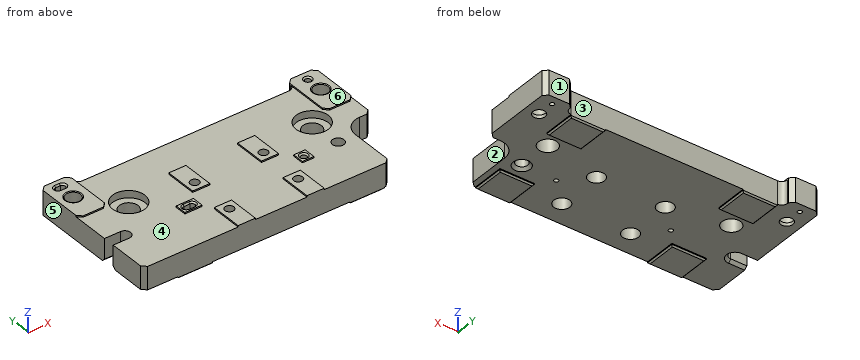
from build123d import *

# Parameters (mm, degrees)
SKETCH1_W                                        = 152.4
SKETCH1_H                                        = 69.85
BASE_EXTRUDE_DEPTH                               = 12.7
SKETCH29_W                                       = 19.05
SKETCH29_H                                       = 17.78
MOUNTING_SURFACES_STAGE2_DEPTH                   = 1.27
CHAMFER1_SIZE                                    = 2.286
SKETCH17_W                                       = 9.525
SKETCH17_H                                       = 17.4625
MOUNTING_SURFACES_MAGNET_BRACKET_DEPTH           = 0.762
EXTRUDE1_DEPTH                                   = 13.462
SKETCH18_R                                       = 1.59512
PIN_HOLES_SLOTS_MAGNET_BLOCK_BOBIN_DEPTH         = 1.762
PIN_HOLES_SLOTS_MAGNET_BLOCK_BOBIN_DEPTH_BACK    = 6.35
SKETCH19_W                                       = 6.35
SKETCH19_H                                       = 6.35
SKETCH19_R                                       = 1.59512
SKETCH19_W_2                                     = 9.525
PIN_HOLE_SLOT_MAGNET_BLOCK_SURFACE_DEPTH         = 0.762
CLEARANCE_CUT_GS_13_SCREW_HEAD_DEPTH             = 1.762
CLEARANCE_CUT_GS_13_SCREW_HEAD_DEPTH_BACK        = 14.97
CBORE_FOR_8_SOCKET_HEAD_CAP_SCREW1_D             = 4.9149
CBORE_FOR_8_SOCKET_HEAD_CAP_SCREW1_CBORE_D       = 8.89
CBORE_FOR_8_SOCKET_HEAD_CAP_SCREW1_CBORE_DEPTH   = 7.62
TAPPED_HOLE_FOR_1_4_20_HELICOIL1_AT_2_COUNT      = 2
TAPPED_HOLE_FOR_1_4_20_HELICOIL1_AT_2_PITCH      = 137.16
SKETCH28_R                                       = 3.18389
PIN_HOLE_SLOT_TO_STAGE2_DEPTH                    = 15.732
CBORE_FOR_3_8_SOCKET_HEAD_CAP_SCREW1_D           = 10.3124
CBORE_FOR_3_8_SOCKET_HEAD_CAP_SCREW1_CBORE_D     = 17.8562
CBORE_FOR_3_8_SOCKET_HEAD_CAP_SCREW1_CBORE_DEPTH = 3.9624
CHAMFER3_SIZE                                    = 0.762
F_3_32_0_09375_DIAMETER_HOLE1_D                  = 2.38125
CHAMFER4_SIZE                                    = 1.524
SKETCH37_W                                       = 15.875
SKETCH37_H                                       = 6.0325
EXTRUDE2_DEPTH                                   = 0.762
FILLET1_R                                        = 3.175
CHAMFER7_SIZE                                    = 0.762
CHAMFER8_SIZE                                    = 2.286


with BuildPart() as part:
    # Sketch1 → Base Extrude (new body)
    with BuildSketch(Plane.XY):
        with Locations((0, 9.525)):
            Rectangle(SKETCH1_W, SKETCH1_H)
    extrude(amount=BASE_EXTRUDE_DEPTH)

    # Sketch29 → Mounting Surfaces_ Stage2 (add)
    with BuildSketch(Plane(origin=(0, 0, 0), x_dir=(-1, 0, 0), z_dir=(0, 0, -1))):
        with Locations((-47.625, 35.56)):
            Rectangle(SKETCH29_W, SKETCH29_H)
        with Locations((-47.625, -16.51)):
            Rectangle(SKETCH29_W, SKETCH29_H)
        with Locations((47.625, 35.56)):
            Rectangle(SKETCH29_W, SKETCH29_H)
        with Locations((47.625, -16.51)):
            Rectangle(SKETCH29_W, SKETCH29_H)
    extrude(amount=MOUNTING_SURFACES_STAGE2_DEPTH)

    # Chamfer1
    chamfer1_edges = [part.edges().sort_by_distance(p)[0] for p in [
        (-76.2, 44.45, 6.35),
        (76.2, 44.45, 6.35),
        (76.2, -25.4, 6.35),
        (-76.2, -25.4, 6.35),
    ]]
    chamfer(chamfer1_edges, length=CHAMFER1_SIZE)

    # Sketch17 → Mounting Surfaces_ Magnet _ Bracket (add)
    with BuildSketch(Plane.XY.offset(12.7)):
        with Locations((-19.05, 16.66875)):
            Rectangle(SKETCH17_W, SKETCH17_H)
        with Locations((19.05, 16.66875)):
            Rectangle(SKETCH17_W, SKETCH17_H)
        with Locations((19.05, -16.66875)):
            Rectangle(SKETCH17_W, SKETCH17_H)
        with Locations((-19.05, -16.66875)):
            Rectangle(SKETCH17_W, SKETCH17_H)
        Polygon((-73.914, 44.45), (-76.2, 42.164), (-76.2, 27.94), (-60.325, 27.94), (-60.325, 44.45), align=None)
        Polygon((73.914, 44.45), (60.325, 44.45), (60.325, 27.94), (76.2, 27.94), (76.2, 42.164), align=None)
    extrude(amount=MOUNTING_SURFACES_MAGNET_BRACKET_DEPTH)

    # Sketch36 → Extrude1 (add)
    with BuildSketch(Plane.XY.offset(13.462)):
        Polygon((-76.2, 42.164), (-76.2, 48.1965), (-73.914, 50.4825), (-60.325, 50.4825), (-60.325, 44.45), (-73.914, 44.45), align=None)
        Polygon((60.325, 44.45), (60.325, 50.4825), (73.914, 50.4825), (76.2, 48.1965), (76.2, 42.164), (73.914, 44.45), align=None)
    extrude(amount=-EXTRUDE1_DEPTH)

    # Sketch18 → Pin holes _ Slots_ Magnet Block _ Bobin (cut, two sides)
    with BuildSketch(Plane.XY.offset(12.7)) as pin_holes_slots_magnet_block_bobin_sk:
        with Locations((31.75, 0)):
            Circle(SKETCH18_R)
        with Locations((68.58, 45.72)):
            Circle(SKETCH18_R)
        with BuildLine():
            Line((-33.3375, 1.59512), (-30.1625, 1.59512))
            ThreePointArc((-30.1625, 1.59512), (-28.56738, 0), (-30.1625, -1.59512))
            Line((-30.1625, -1.59512), (-33.3375, -1.59512))
            ThreePointArc((-33.3375, -1.59512), (-34.93262, 0), (-33.3375, 1.59512))
        make_face()
        with BuildLine():
            Line((-69.85, 47.31512), (-67.31, 47.31512))
            ThreePointArc((-67.31, 47.31512), (-65.71488, 45.72), (-67.31, 44.12488))
            Line((-67.31, 44.12488), (-69.85, 44.12488))
            ThreePointArc((-69.85, 44.12488), (-71.44512, 45.72), (-69.85, 47.31512))
        make_face()
    extrude(amount=PIN_HOLES_SLOTS_MAGNET_BLOCK_BOBIN_DEPTH, mode=Mode.SUBTRACT)
    extrude(pin_holes_slots_magnet_block_bobin_sk.sketch, amount=-PIN_HOLES_SLOTS_MAGNET_BLOCK_BOBIN_DEPTH_BACK, mode=Mode.SUBTRACT)

    # Sketch19 → Pin hole _ Slot_ Magnet Block surface (add)
    with BuildSketch(Plane.XY.offset(12.7)):
        with Locations((31.75, 0)):
            Rectangle(SKETCH19_W, SKETCH19_H)
        with Locations((31.75, 0)):
            Circle(SKETCH19_R, mode=Mode.SUBTRACT)
        with Locations((-31.75, 0)):
            Rectangle(SKETCH19_W_2, SKETCH19_H)
        with BuildLine():
            Line((-30.1625, 1.59512), (-33.3375, 1.59512))
            ThreePointArc((-33.3375, 1.59512), (-34.93262, 0), (-33.3375, -1.59512))
            Line((-33.3375, -1.59512), (-30.1625, -1.59512))
            ThreePointArc((-30.1625, -1.59512), (-28.56738, 0), (-30.1625, 1.59512))
        make_face(mode=Mode.SUBTRACT)
    extrude(amount=PIN_HOLE_SLOT_MAGNET_BLOCK_SURFACE_DEPTH)

    # Sketch20 → Clearance Cut_ GS-13 Screw Head (cut, two sides)
    with BuildSketch(Plane.XY.offset(12.7)) as clearance_cut_gs_13_screw_head_sk:
        with BuildLine():
            Line((60.325, 0), (60.325, -25.4))
            Line((60.325, -25.4), (73.914, -25.4))
            Line((73.914, -25.4), (76.2, -23.114))
            Line((76.2, -23.114), (76.2, 9.525))
            Line((76.2, 9.525), (69.85, 9.525))
            ThreePointArc((69.85, 9.525), (63.114807909, 6.735192091), (60.325, 0))
        make_face()
    extrude(amount=CLEARANCE_CUT_GS_13_SCREW_HEAD_DEPTH, mode=Mode.SUBTRACT)
    extrude(clearance_cut_gs_13_screw_head_sk.sketch, amount=-CLEARANCE_CUT_GS_13_SCREW_HEAD_DEPTH_BACK, mode=Mode.SUBTRACT)

    # CBORE for _8 Socket Head Cap Screw1 (through all)
    with Locations(Plane(origin=(0, 0, 0), x_dir=(-1, 0, 0), z_dir=(0, 0, -1))):
        with Locations((-19.05, 12.7), (19.05, 12.7), (19.05, -12.7), (-19.05, -12.7)):
            CounterBoreHole(CBORE_FOR_8_SOCKET_HEAD_CAP_SCREW1_D / 2, CBORE_FOR_8_SOCKET_HEAD_CAP_SCREW1_CBORE_D / 2, CBORE_FOR_8_SOCKET_HEAD_CAP_SCREW1_CBORE_DEPTH)

    # Sketch25 → Tapped Hole for 1_4-20 Helicoil1 (revolve, cut)
    with BuildSketch(Plane(origin=(68.58, 36.195, 13.462), x_dir=(0, -1, 0), z_dir=(1, 0, 0))):
        Polygon((0, 0), (0, 14.732025), (3.3782, 14.732025), (3.3782, 11.6586), (4.04749, 11.6586), (4.04749, 0.30282599), (4.572, 0), align=None)
    tapped_hole_for_1_4_20_helicoil1 = revolve(axis=Axis((68.58, 36.195, 19.812), (0, 0, -1)), mode=Mode.SUBTRACT)

    # Tapped Hole for 1_4-20 Helicoil1 at 2: Tapped Hole for 1_4-20 Helicoil1 ×2
    with Locations(*[(-i * TAPPED_HOLE_FOR_1_4_20_HELICOIL1_AT_2_PITCH, 0, 0) for i in range(1, TAPPED_HOLE_FOR_1_4_20_HELICOIL1_AT_2_COUNT)]):
        add(tapped_hole_for_1_4_20_helicoil1, mode=Mode.SUBTRACT)

    # Sketch28 → Pin Hole _ Slot to Stage2 (cut, through all)
    with BuildSketch(Plane(origin=(0, 0, -1.27), x_dir=(-1, 0, 0), z_dir=(0, 0, -1))):
        with Locations(Location((-50.8, 0, 0), (0, 0, 180))):  # turned: the seam where the file's is
            Circle(SKETCH28_R)
        with BuildLine():
            Line((67.31, 3.18389), (80.01, 3.18389))
            ThreePointArc((80.01, 3.18389), (83.19389, 0), (80.01, -3.18389))
            Line((80.01, -3.18389), (67.31, -3.18389))
            ThreePointArc((67.31, -3.18389), (64.12611, 0), (67.31, 3.18389))
        make_face()
    extrude(amount=-PIN_HOLE_SLOT_TO_STAGE2_DEPTH, mode=Mode.SUBTRACT)

    # CBORE for 3_8 Socket Head Cap Screw1 (through all)
    with Locations(Plane.XY.offset(12.7)):
        with Locations((-50.8, 19.05), (50.8, 19.05)):
            CounterBoreHole(CBORE_FOR_3_8_SOCKET_HEAD_CAP_SCREW1_D / 2, CBORE_FOR_3_8_SOCKET_HEAD_CAP_SCREW1_CBORE_D / 2, CBORE_FOR_3_8_SOCKET_HEAD_CAP_SCREW1_CBORE_DEPTH)

    # Chamfer3
    chamfer3_edges = [part.edges().sort_by_distance(p)[0] for p in [
        (66.98488, 45.72, 13.462),
        (-71.44512, 45.72, 13.462),
        (-68.58, 44.12488, 13.462),
        (-65.71488, 45.72, 13.462),
        (-68.58, 47.31512, 13.462),
        (30.15488, 0, 13.462),
        (-31.75, 1.59512, 13.462),
        (-28.56738, 0, 13.462),
        (-31.75, -1.59512, 13.462),
        (-34.93262, 0, 13.462),
    ]]
    chamfer(chamfer3_edges, length=CHAMFER3_SIZE)

    # 3_32 _0.09375_ Diameter Hole1 (through all)
    with Locations(Plane(origin=(0, 0, -1.27), x_dir=(-1, 0, 0), z_dir=(0, 0, -1))):
        with Locations((68.58, 45.72), (-68.58, 45.72), (-31.75, 0), (31.75, 0)):
            Hole(F_3_32_0_09375_DIAMETER_HOLE1_D / 2)

    # Chamfer4
    chamfer4_edges = [part.edges().sort_by_distance(p)[0] for p in [
        (47.61611, 0, 0),
        (-64.12611, 0, 0),
        (-71.755, 3.18389, 0),
        (-71.755, -3.18389, 0),
    ]]
    chamfer(chamfer4_edges, length=CHAMFER4_SIZE)

    # Sketch37 → Extrude2 (add)
    with BuildSketch(Plane.XY.offset(13.462)):
        with Locations((-68.2625, 24.92375)):
            Rectangle(SKETCH37_W, SKETCH37_H)
        with Locations((68.2625, 24.92375)):
            Rectangle(SKETCH37_W, SKETCH37_H)
    extrude(amount=-EXTRUDE2_DEPTH)

    # Fillet1
    fillet1_edges = [part.edges().sort_by_distance(p)[0] for p in [
        (60.325, 44.45, 6.35),
        (-60.325, 44.45, 6.35),
    ]]
    fillet(fillet1_edges, radius=FILLET1_R)

    # Chamfer7
    chamfer7_edges = [part.edges().sort_by_distance(p)[0] for p in [
        (-47.625, 44.45, -1.27),
        (-57.15, 35.56, -1.27),
        (-47.625, 26.67, -1.27),
        (-38.1, 35.56, -1.27),
        (47.625, 44.45, -1.27),
        (38.1, 35.56, -1.27),
        (47.625, 26.67, -1.27),
        (57.15, 35.56, -1.27),
        (47.625, -25.4, -1.27),
        (57.15, -16.51, -1.27),
        (47.625, -7.62, -1.27),
        (38.1, -16.51, -1.27),
        (-47.625, -25.4, -1.27),
        (-38.1, -16.51, -1.27),
        (-47.625, -7.62, -1.27),
        (-57.15, -16.51, -1.27),
    ]]
    chamfer(chamfer7_edges, length=CHAMFER7_SIZE)

    # Chamfer8
    chamfer8_edges = [part.edges().sort_by_distance(p)[0] for p in [
        (-60.325, 50.4825, 6.731),
        (60.325, 50.4825, 6.731),
        (60.325, -25.4, 6.35),
        (76.2, 9.525, 6.35),
        (-76.2, 21.9075, 13.081),
        (-60.325, 21.9075, 13.081),
        (60.325, 21.9075, 13.081),
        (76.2, 21.9075, 13.081),
    ]]
    chamfer(chamfer8_edges, length=CHAMFER8_SIZE)


solid = part.part
Can you work these out from the model? Positions are in its coordinate system, mm. Face numbers are marked on the shaded views. A direction names the side the tool comes from. Coordinates: 2 decimals unless noted, no trailing zeros. Order: outer loops, then holes, each group sorted by start corner. A loop starts at its lowest first (then second) coordinate and runs counter-clockwise, first axis right, second up. Notation, with made-up numbers: (80, -14.5) - (133, -14.5) arc R25 cw to (133, 10.5) - close; hole circle Ø1 at (71, -35). An arc over 180 degrees is marked (long way). Answer as a JSON object with one key per item and string values. Group by question number.
Q1. I need wall thicknesses on line 1 (X direction, y = -12.5, z = 3.25) (1 decimal); line 2 (Y direction, x = 50.8, z = 9.75); line 3 (Y direction, x = 19.05, z = 4.5) (3 decimals). Which ranges of each line are inside material? Lowest first, please. Write a range as from..to.
Q2. Imagine slicing it at A-A (y = 19.05). Please give me the cut outline in (x, z), and give its area (3 significant figures).
Q3. On a 3-axis mill with a long thin cutter (end or side, diameter ignored), from which of +Z, -Z, +X, -X, +Y, -Y can I reach the whole of each face in a straight line? I mean the marked faces 1 and 2. Say none if no direction works.
Q4. Will these pins go through, and if not, where does the flat tip stop? P1, Ø2.5, axis at x = 21, y = 14.5, coming from the -Z side; P2, Ø1.5, axis at x = -57, y = 2.5, coming from the -Z side; P3, Ø2, axis at x = -36.5, z = 12, coming from the +Y side.
Q5. Imagine slicing it at D-D (x = -53). Please give me the cut outline in (y, z).
Q6. We'd pull the mould along X, two halves only. Please class the marked faces 3, 4, 5 and 6: +X half, -X half, draft (parallel to the pull), parting line (faces both ways), or undercut.
Q7. Imagine slicing it at B-B (x = -19.05). Give the number of separate pieces and of enclosed holes in the cut face, and give its area (3 significant figures).
Determined:
{
 "1": {"line 1": "x = -76.2..-23.5, -14.6..14.6, 23.5..60.3", "line 2": "y = -25.4..-3.18, 3.18..10.12, 27.98..44.45", "line 3": "y = -25.4..-17.145, -8.255..8.255, 17.145..44.45"},
 "2": {"outline": "(-76.2, 0) - (-55.96, 0) - (-55.96, 8.74) - (-59.73, 8.74) - (-59.73, 12.7) - (-76.2, 12.7) - close; (-45.64, 0) - (45.64, 0) - (45.64, 8.74) - (41.87, 8.74) - (41.87, 12.7) - (23.81, 12.7) - (23.81, 13.46) - (14.29, 13.46) - (14.29, 12.7) - (-14.29, 12.7) - (-14.29, 13.46) - (-23.81, 13.46) - (-23.81, 12.7) - (-41.87, 12.7) - (-41.87, 8.74) - (-45.64, 8.74) - close; (55.96, 0) - (76.2, 0) - (76.2, 12.7) - (59.73, 12.7) - (59.73, 8.74) - (55.96, 8.74) - close", "area": "1,630 mm2"},
 "3": {"face 1": "+Z, -Z, +X, -X, +Y", "face 2": "+Z, -Z, +X, -Y"},
 "4": {"P1": "stops at z = 7.62", "P2": "stops at z = 0", "P3": "stops at y = 44.45"},
 "5": {"outline": "(-25.4, -0.51) - (-24.64, -1.27) - (-8.38, -1.27) - (-7.62, -0.51) - (-7.62, 0) - (14.39, 0) - (14.39, 8.74) - (10.4, 8.74) - (10.4, 12.7) - (-25.4, 12.7) - close; (23.71, 0) - (26.67, 0) - (26.67, -0.51) - (27.43, -1.27) - (43.69, -1.27) - (44.45, -0.51) - (44.45, 12.7) - (27.7, 12.7) - (27.7, 8.74) - (23.71, 8.74) - close"},
 "6": {"face 3": "undercut", "face 4": "undercut", "face 5": "-X half", "face 6": "draft"},
 "7": {"separate pieces": "3", "enclosed holes": "0", "area": "721 mm2"}
}
